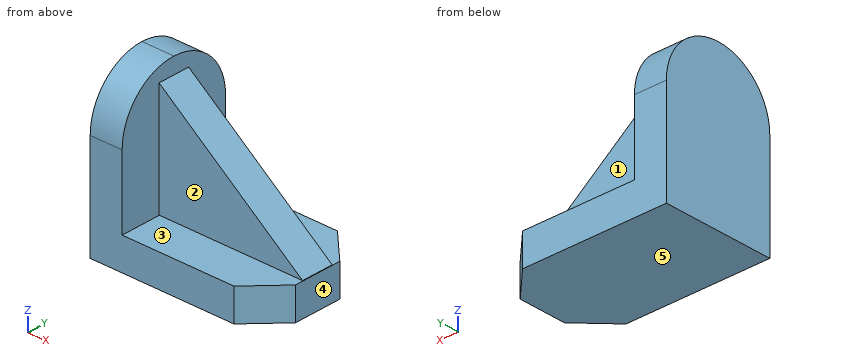
Autodesk Fusion 360 part; units mm, degrees
sketch "Sketch1" plane through (0, 0, 0) normal (0, 0, 1) x (1, 0, 0)
  line L0 (33, -21) -> (-33, -21)
  line L1 (-33, -21) -> (-33, 21)
  line L2 (-33, 21) -> (33, 21)
  line L3 (33, 21) -> (33, -21)
  line L4 (33, -21) -> (-33, 21) construction
  line L5 (-33, -21) -> (33, 21) construction
  dimension "d1" = 66
  dimension "d2" = 42
extrude "Extrude1" add sketch "Sketch1" along normal blind 12
chamfer "Chamfer1" distance 12 angle 45 2 edges at (33, -21, 6) (33, 21, 6)
sketch "Sketch2" plane through (0, 0, 12) normal (0, 0, 1) x (-1, 0, 0)
  line L0 (-33, -9) -> (-21, -21)
  line L1 (-21, -21) -> (33, -21)
  line L2 (33, -21) -> (33, 21)
  line L3 (33, 21) -> (-21, 21)
  line L4 (-21, 21) -> (-33, 9)
  line L5 (-33, 9) -> (-33, -9)
  line L6 (33, -21) -> (21, -21)
  line L7 (21, -21) -> (21, 21)
  line L8 (21, 21) -> (33, 21)
  line L9 (33, 21) -> (33, -21)
  dimension "d6" = 12
extrude "Extrude2" add sketch "Sketch2" along normal blind 48 contours L1 L2 L3 L6 L7 L8 L9
fillet "Fillet1" radius 21 2 edges at (-27, -21, 60) (-27, 21, 60)
sketch "Sketch3" plane through (0, 0, 0) normal (0, 1, 0) x (1, 0, 0)
  line L0 (-21.1039, -54.093) -> (-21.1039, -12.093)
  line L1 (-21.1039, -12.093) -> (32.8961, -12.093)
  line L2 (32.8961, -12.093) -> (-21.1039, -54.093)
  dimension "d10" = 42
  dimension "d11" = 54
extrude "Extrude3" add sketch "Sketch3" along normal mid plane 12
equation "d7 = 60 mm - 12 mm"
equation "d11 = 66 mm - 12 mm"
Source: CAD feature listing. Evaluate the final solid. Frame: model axes, mm. Face numbers are marked on the shaded views. A direction names the side the tool comes from. Round coordinates to 2 decimals unless told otherwise and drop trailing zeros. Loops run counter-clockwise (first coordinate to the right, second up) from the corner with the lowest first, then second, coordinate; pieces in that order, holes last. Notation, with made-up numbers: M 38,-5.75 L 88,-5.75 A17 ccw 88,24.25 Z; hole C -39,67 d6. An arc over 180 degrees is marked long. Use a Markdown table: item, result. Add a question column.
1. Cut plane C-C, the plane y = -2.5. Output: boundary loops of the cut face in (x, z), and give its area (3 significant figures).
2. Set-up query: the marked faces 1, 2, 3, 4 and 5. Return all of +Z, -Z, +X, -X, +Y, -Y with unobstructed straight access to the full face (end or side cutting, diameter ignored); none if empty.
3. Ray query, line 1 along Z through (x, y) = (-17, 8.5); line 2 along X through (y, z) = (11, 38); line 3 along Y through (x, z) = (9.5, 26). Return the intervals inside material, ascending. Write a range as [from, to].
4. Contact query for flat-ended pins moving along their axis: pin 1 (6 mm diameter, centred on y = 16, z = 9, fed in from +X); pin 2 (21 mm diameter, centred on x = 3, y = 10, fed in from +Z); pin 3 (8 mm diameter, centred on y = 2, z = 43, fed in from +X); pin 4 (2 mm diameter, centred on x = 4, z = 37, fed in from +Y). Output: stop coordinate, or through.
5. Cut plane A-A, the plane z = 11. Output: boundary loops of the cut face in (x, y), and give its area (3 significant figures).
6. Cut plane B-B, the plane x = -3. Output: boundary loops of the cut face in (y, z), and give its area (3 significant figures).
Solution:
| question | item | result |
|---|---|---|
| 1 | outline | M -33,0 L 33,0 L 33,12 L -21,12 L -21,12.09 L 32.9,12.09 L -21,54.01 L -21,59.85 L -33,59.85 Z |
| 1 | area | 2,500 mm2 |
| 2 | face 1 | +Z, +X, +Y |
| 2 | face 2 | +Z, +X, -Y |
| 2 | face 3 | +X, +Y, -Y |
| 2 | face 4 | +Z, -Z, +X, +Y, -Y |
| 2 | face 5 | -Z, +X, -X, +Y, -Y |
| 3 | line 1 | z = [0, 12] |
| 3 | line 2 | x = [-33, -21] |
| 3 | line 3 | y = [-6, 6] |
| 4 | pin 1 | stops at x = 29 |
| 4 | pin 2 | stops at z = 42.9 |
| 4 | pin 3 | stops at x = -1.7 |
| 4 | pin 4 | passes through |
| 5 | outline | M -33,-21 L 21,-21 L 33,-9 L 33,9 L 21,21 L -33,21 Z |
| 5 | area | 2,630 mm2 |
| 6 | outline | M -21,0 L 21,0 L 21,12 L -21,12 Z; M -6,12.09 L 6,12.09 L 6,40.01 L -6,40.01 Z |
| 6 | area | 839 mm2 |
